Autodesk Inventor part; units mm, degrees
ref_plane "YZ Plane" through (0, 0, 0) normal (1, 0, 0) x (0, 1, 0)
ref_plane "XZ Plane" through (0, 0, 0) normal (0, 1, 0) x (-1, 0, 0)
ref_plane "XY Plane" through (0, 0, 0) normal (0, 0, 1) x (1, 0, 0)
sketch "スケッチ1" plane through (0, 0, 0) normal (0, 0, 1) x (1, 0, 0)
  circle A0 centre (0, 0) radius 4.05
  circle A1 centre (0, 0) radius 11.5
  line L0 (-1.2, 1.6) -> (1.2, 1.6)
  line L1 (11.3882, 1.6) -> (1.2, 1.6)
  line L2 (-1.2, 1.6) -> (-11.3882, 1.6)
  circle A2 centre (0, 0) radius 2
  line L3 (9.1241, -7) -> (-9.1241, -7)
  point P0 (3.7206, 1.6)
  point P1 (-3.7206, 1.6)
  dimension "d0" = 8.1
  dimension "d1" = 23
  dimension "d3" = 4
  dimension "d4" = 2.4
  dimension "d5" = 7
extrude "押し出し1" add sketch "スケッチ1" along normal blind 12 contours A0 L1 A1 L3 L2
sketch "スケッチ3" plane through (-11.3882, 1.6, 0) normal (0, 1, 0) x (1, 0, 0)
  line L0 (22.7763, 0) -> (15.1087, 0)
  line L1 (7.6676, 0) -> (0, 0)
  point P0 (11.3882, 0)
  point P1 (3.8882, -6)
  point P2 (18.8882, -6)
  dimension "d8" = 6
  dimension "d9" = 7.5
  dimension "d10" = 7.5
  dimension "d11" = 6
hole "穴1" at (-7.5, 1.6, 6) at (7.5, 1.6, 6) direction (0, -1, 0) diameter 3.4 end through all
properties part number "SU22_3DP_EU_Sub_sn" material "ABS プラスチック"
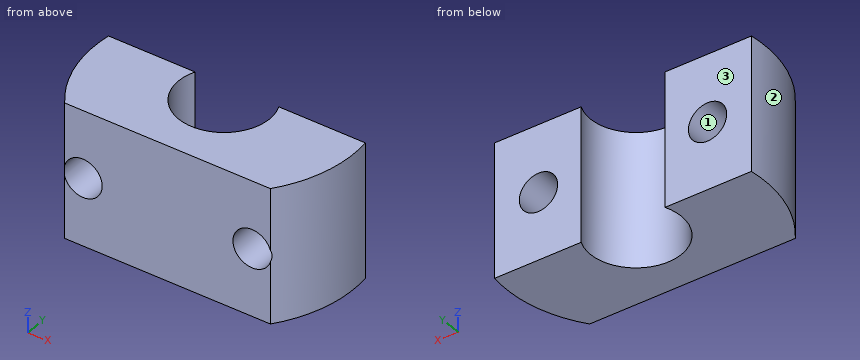
Here's how the part is built. I have some questions about the finished solid (model axes, mm). Face numbers are marked on the shaded views. Give positions to 0.01 mm unless a question says otherwise; leave off trailing zeros. Loops run counter-clockwise (first coordinate to the right, second up) from the corner with the lowest first, then second, coordinate; pieces in that order, holes last. Notation, with made-up numbers: (65, 80) -> (119, 80) arc R32 cw to (119, 113) -> close; hole circle Ø7 at (10.25, -32). An arc over 180 degrees is marked (long way). Use one line per item in the form item = value. Start each with the question number.
1) For P1, Ø1, axis at y = -1, z = 4, coming from the -X side; P2, Ø2, axis at x = 7.5, z = 6, coming from the +Y side, each with a flat end and sliding along its axis, tell me the tip position at first contact or that it passes through.
2) Please list where these lines run through material, in increasing order: line 1 along X through (y, z) = (-0.5, 7); line 2 along X through (y, z) = (-2, 7.5); line 3 along X through (y, z) = (-5.5, 5.25).
3) Imagine slicing it at D-D (y = -2). Please give me the cut outline in (x, z), then the cut area to 3 significant figures.
4) Imagine slicing it at A-A (y = 0). Please give me the cut outline in (x, z).
5) Imagine slicing it at C-C (z = 6). Please give me the cut outline in (x, y).
6) Thinking about a two-plate mould opening in X: for the marked faces 1, 2 and 3, which applies, +X half, -X half, draft (parallel to the pull), parting line (faces both ways), or undercut?
7) Imagine slicing it at B-B (x = -7.5). Please give me the cut outline in (y, z), then the cut area to 3 significant figures.
Check values:
q1.P1 = -11.49
q1.P2 = through
q2.line_1 = -11.49 to -8.87, -6.13 to -4.02, 4.02 to 6.13, 8.87 to 11.49
q2.line_2 = -11.32 to -8.3, -6.7 to -3.52, 3.52 to 6.7, 8.3 to 11.32
q2.line_3 = -10.1 to -9.03, -5.97 to 5.97, 9.03 to 10.1
q3.outline = (-11.32, 0) -> (-3.52, 0) -> (-3.52, 12) -> (-11.32, 12) -> close; (3.52, 0) -> (11.32, 0) -> (11.32, 12) -> (3.52, 12) -> close; hole circle Ø3.4 at (-7.5, 6); hole circle Ø3.4 at (7.5, 6)
q3.area = 169 mm^2
q4.outline = (-11.5, 0) -> (-4.05, 0) -> (-4.05, 12) -> (-11.5, 12) -> close; (4.05, 0) -> (11.5, 0) -> (11.5, 12) -> (4.05, 12) -> close; hole circle Ø3.4 at (-7.5, 6); hole circle Ø3.4 at (7.5, 6)
q5.outline = (-11.39, 1.6) arc R11.5 ccw to (-9.2, -6.9) -> (-9.2, 1.6) -> close; (-5.8, -7) -> (5.8, -7) -> (5.8, 1.6) -> (3.72, 1.6) arc R4.05 cw (long way) to (-3.72, 1.6) -> (-5.8, 1.6) -> close; (9.2, -6.9) arc R11.5 ccw to (11.39, 1.6) -> (9.2, 1.6) -> close
q6.face_1 = undercut
q6.face_2 = -X half
q6.face_3 = draft
q7.outline = (-7, 0) -> (1.6, 0) -> (1.6, 4.3) -> (-7, 4.3) -> close; (-7, 7.7) -> (1.6, 7.7) -> (1.6, 12) -> (-7, 12) -> close
q7.area = 74.0 mm^2
